from build123d import *

# Parameters (mm, degrees)
F0_R     = 2.75
F1_DEPTH = 1.825
F3_COUNT = 8
F4_DEPTH = 3.775
F6_DEPTH = 7.551


with BuildPart() as f1:
    # F0 (on Front) → F1 (new body, symmetric)
    with BuildSketch(Plane.XZ):
        with BuildLine():
            add(Edge.make_bspline(
                [(0.5, 4.6481851297), (0.5992553827, 4.3830381396), (0.8018424102, 3.8418549905), (0.7012885529, 3.2371652786), (0.65, 2.9287369291)],
                knots=[0, 0, 0, 0, 0.489939479, 1, 1, 1, 1], degree=3))
            ThreePointArc((0.5, 4.6481851297), (0, 4.675), (-0.5, 4.6481851297))
            add(Edge.make_bspline(
                [(-0.5, 4.6481851297), (-0.5992553827, 4.3830381396), (-0.8018424102, 3.8418549905), (-0.7012885529, 3.2371652786), (-0.65, 2.9287369291)],
                knots=[0, 0, 0, 0, 0.489939479, 1, 1, 1, 1], degree=3))
            ThreePointArc((-0.65, 2.9287369291), (0, 3), (0.65, 2.9287369291))
        make_face()
        with BuildLine():
            ThreePointArc((3, 0), (2.3398717914, 1.8774983356), (0.65, 2.9287369291))
            ThreePointArc((0.65, 2.9287369291), (0, 3), (-0.65, 2.9287369291))
            ThreePointArc((-0.65, 2.9287369291), (-1.8774983356, -2.3398717914), (3, 0))
        make_face()
        Circle(F0_R, mode=Mode.SUBTRACT)
    extrude(amount=F1_DEPTH, both=True)

    # F3: F1 ×8 about axis
    f3_axis = Axis((0, -1.825, 0), (0, -1, 0))


with BuildPart() as f1_1:
    add(f1.part)
    for i in range(1, F3_COUNT):
        add(f1.part.rotate(f3_axis, i * 360 / F3_COUNT))

    # F0 (on Front) → F4 (join, symmetric)
    with BuildSketch(Plane.XZ):
        Circle(F0_R)
    extrude(amount=F4_DEPTH, both=True)

    # F5 (on face) → F6 (cut, through all)
    with BuildSketch(Plane.XZ.offset(3.775)):
        with BuildLine():
            ThreePointArc((2.3313088598, -0.9), (2.4567195445, -0.4577445572), (2.499, 0))
            ThreePointArc((2.499, 0), (2.4567195445, 0.4577445572), (2.3313088598, 0.9))
            Line((2.3313088598, 0.9), (0.9, 0.9))
            Line((0.9, 0.9), (0.9, 2.3313088598))
            ThreePointArc((0.9, 2.3313088598), (0, 2.499), (-0.9, 2.3313088598))
            Line((-0.9, 2.3313088598), (-0.9, 0.9))
            Line((-0.9, 0.9), (-2.3313088598, 0.9))
            ThreePointArc((-2.3313088598, 0.9), (-2.499, 0), (-2.3313088598, -0.9))
            Line((-2.3313088598, -0.9), (-0.9, -0.9))
            Line((-0.9, -0.9), (-0.9, -2.3313088598))
            ThreePointArc((-0.9, -2.3313088598), (0, -2.499), (0.9, -2.3313088598))
            Line((0.9, -2.3313088598), (0.9, -0.9))
            Line((0.9, -0.9), (2.3313088598, -0.9))
        make_face()
    extrude(amount=-F6_DEPTH, mode=Mode.SUBTRACT)


solid = f1_1.part
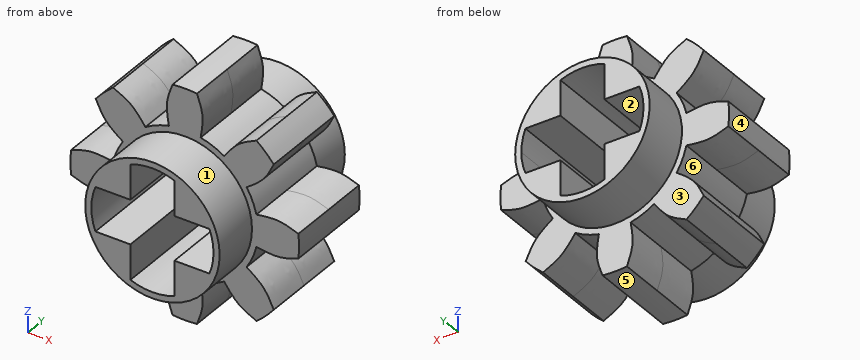
Input: part model. Units: mm. Frame: model coordinates. Face numbers are marked on the shaded views. A direction names the side the tool comes from. Give positions to 0.01 mm unless a question says otherwise; leave off trailing zeros. Order: outer loops, then holes, each group sorted by start corner. A loop starts at its lowest first (then second) coordinate and runs counter-clockwise, first axis right, second up. Notation, with made-up numbers: (50.25, 3.5) -> (65.25, 3.5) arc R14 ccw to (65.25, 11.5) -> close; hole circle Ø10 at (42.5, 75.25). An arc over 180 degrees is marked (long way). Use one line per item in the form item = value.
1) Reachability of the marked faces 1, 2 and 3 from +Z, -Z, +X, -X, +Y, -Y: full face, straight path, thin tool, end or side. Return the list, or none.
Response values:
face_1 = -Y
face_2 = +Y, -Y
face_3 = +Y
2) Section A-A, the plane x = 0. Return loops of the section in (y, z) (3 decimals).
Response values:
outline = (-3.775, -2.75) -> (-1.825, -2.75) -> (-1.825, -4.675) -> (1.825, -4.675) -> (1.825, -2.75) -> (3.775, -2.75) -> (3.775, -2.499) -> (-3.775, -2.499) -> close; (-3.775, 2.499) -> (3.775, 2.499) -> (3.775, 2.75) -> (1.825, 2.75) -> (1.825, 4.675) -> (-1.825, 4.675) -> (-1.825, 2.75) -> (-3.775, 2.75) -> close
3) Section C-C, the plane x = 3.25. Count the separate pieces of the cut face and the enclosed holes in it, and give its area (3 significant figures).
Response values:
separate_pieces = 3
enclosed_holes = 0
area = 13.4 mm^2
4) First-contact query: pin 1 Ø1 at (y, z) = (-2.5, 3) entering from +X; pin 2 Ø0.7 at (y, z) = (-1, 1.5) entering from +X; pin 3 Ø0.7 at (y, z) = (0, -1.5) entering from -X. Flat tips, straight axial feed; report the tip coordinate or a pass-through.
Response values:
pin_1 = 1.15
pin_2 = 2.85
pin_3 = -2.85
5) Section B-B, the plane y = -2.5. Return loops of the section in (x, z).
Response values:
outline = circle Ø5.5 at (0, 0); hole (-2.33, -0.9) -> (-0.9, -0.9) -> (-0.9, -2.33) arc R2.5 ccw to (0.9, -2.33) -> (0.9, -0.9) -> (2.33, -0.9) arc R2.5 ccw to (2.33, 0.9) -> (0.9, 0.9) -> (0.9, 2.33) arc R2.5 ccw to (-0.9, 2.33) -> (-0.9, 0.9) -> (-2.33, 0.9) arc R2.5 ccw to start
6) Line query: probe 1 along Z at (x, y) = (3.25, 0.5); probe 2 along Z at (x, y) = (-3, -1.5). Output: solid intervals per line, ascending.
Response values:
probe_1 = -3.36 to -2.23, -0.7 to 0.7, 2.23 to 3.36
probe_2 = -3.59 to -1.97, -0.66 to 0.66, 1.97 to 3.59
7) Mould query, pull axis Z, two halves, no side actions, for the marked faces 4, 5 and 6. Classes: pulls with the +Z half, pulls with the -Z half, needs draft (parallel to the pull), parting line crosses it, or undercut.
Response values:
face_4 = parting line crosses it
face_5 = pulls with the -Z half
face_6 = undercut
